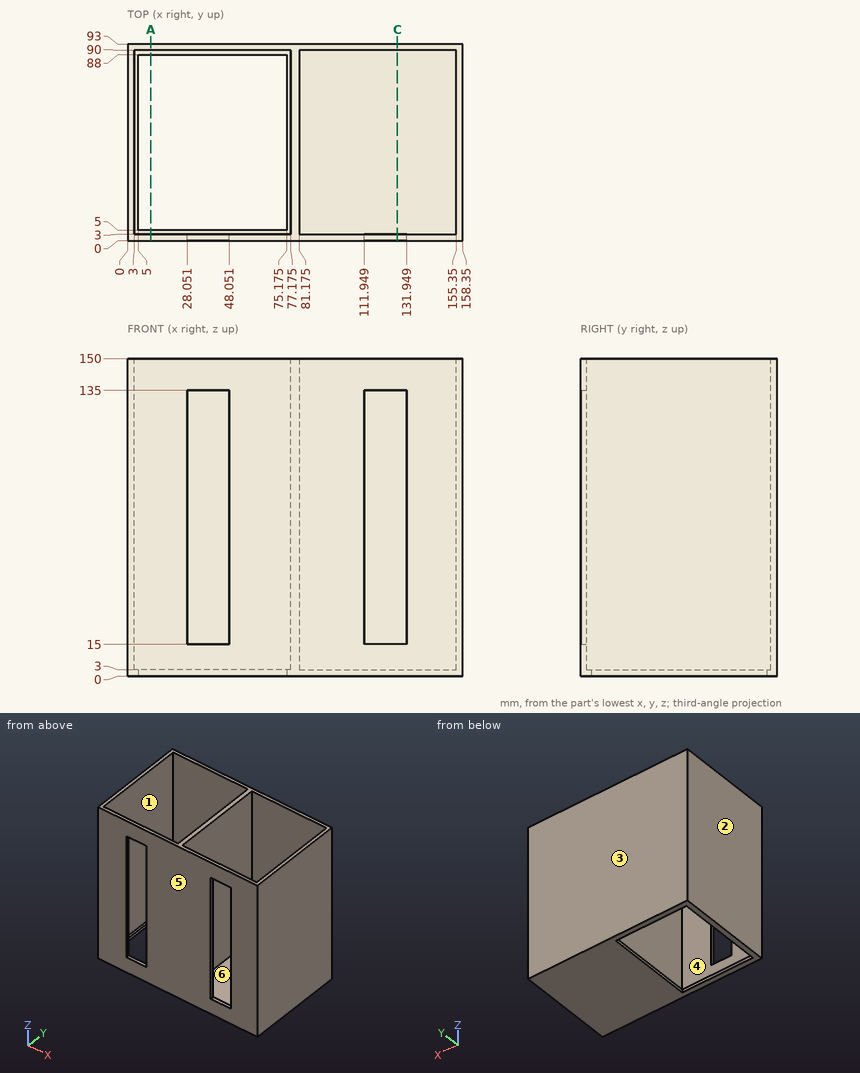
Job drawing, mm, ordinate dimensions from the low corner. One solid piece. A direction names the side the tool comes from. Give positions to 0.01 mm unless a question says otherwise; leave off trailing zeros. Loops run counter-clockwise (first coordinate to the right, second up) from the corner with the lowest first, then second, coordinate; pieces in that order, holes last. Notation, with made-up numbers: M 4.5,68 L 19.5,68 A22 cw 19.5,99 Z; hole C -13,55.25 d5. An arc over 180 degrees is marked long. Use one line per item in the form item = value.
Item 1: Slice it at A-A on x = 11. List the corners of the cut face in (y, z).
Filled in:
outline = M 0,0 L 5,0 L 5,3 L 3,3 L 3,150 L 0,150 Z; M 88,0 L 93,0 L 93,150 L 90,150 L 90,3 L 88,3 Z
Item 2: Flat gauge pin, fed straight in: pin 1 Ø10 at (x, y) = (124, 14.5) entering from +Z. Where does the tip first touch, or does it go through?
Filled in:
pin_1 = 3
Item 3: Slice it at C-C on x = 127.5. List the corners of the cut face in (y, z).
Filled in:
outline = M 0,0 L 93,0 L 93,150 L 90,150 L 90,3 L 3,3 L 3,15 L 0,15 Z; M 0,135 L 3,135 L 3,150 L 0,150 Z
Item 4: Two-plate mould, pull along Y, no slides. Class the marked faces 1, 2, 3 and 4: released by +Y, released by -Y, zero draft, split by the parting line, or undercut.
Filled in:
face_1 = undercut
face_2 = zero draft
face_3 = released by +Y
face_4 = undercut
Item 5: Drill centre lines: L1, parallel to Y at x = 24, z = 38; L2, parallel to Y at x = 42.5, z = 70.5; L3, parallel to Z at x = 85, y = 49. Where is each one in solid material? Low to high.
Filled in:
L1 = 0 to 3, 90 to 93
L2 = 90 to 93
L3 = 0 to 3
Item 6: Which spindle directions (+Z, -Z, +X, -X, +Y, -Y) get a long thin tool onto all of the face, cutting with end or side? Do the marked faces 5 and 6. Say none if no direction does.
Filled in:
face_5 = +Z, -Z, +X, -X, -Y
face_6 = +Z
